from build123d import *

# Parameters (mm, degrees)
BOSS_EXTRUDE1_DEPTH = 5
CUT_EXTRUDE2_DEPTH  = 714.328929729


with BuildPart() as part:
    # Sketch1 → Boss-Extrude1 (new body)
    with BuildSketch(Plane(origin=(-68.393987025, -9.003975274, 13.699403605), x_dir=(0.23308919144115517, -0.5341135383088325, 0.8126451605888809), z_dir=(0.972455360843524, 0.1280224242624249, -0.19478406005796045))):
        Polygon((290.734459145, 269.471566891), (290.734459145, 334.44233671), (415.531866377, 494.175733816), (509.260454317, 494.175733816), (509.260454317, 469.175733816), (446.760454317, 469.175733816), align=None)
    extrude(amount=BOSS_EXTRUDE1_DEPTH)

    # Sketch3 → Cut-Extrude2 (cut, through all)
    with BuildSketch(Plane(origin=(-63.53171022, -8.363863152, 12.725483305), x_dir=(-0.193117751863984, -0.025423689104136546, -0.9808461499885377), z_dir=(0.9724553608435241, 0.1280224242624253, -0.19478406005796034))):
        Polygon((-103.20824521, -577.778495346), (-102.919185311, -573.588454251), (-98.928669982, -573.863749393), (-98.811669547, -572.167780379), (-96.018308817, -572.360486979), (-96.135309253, -574.056455993), (-86.159020932, -574.74469385), (-86.448080832, -578.934734944), (-96.424369152, -578.246497088), (-96.541369588, -579.942466102), (-99.334730318, -579.749759503), (-99.217729882, -578.053790488), align=None)
        Polygon((-94.487300279, -451.364843062), (-94.19824038, -447.174801967), (-90.207725052, -447.45009711), (-90.090724616, -445.754128095), (-87.297363886, -445.946834695), (-87.414364322, -447.64280371), (-77.438076001, -448.331041566), (-77.727135901, -452.521082661), (-87.703424221, -451.832844804), (-87.820424657, -453.528813819), (-90.613785387, -453.336107219), (-90.496784951, -451.640138205), align=None)
        Polygon((-130.671777813, -684.777132582), (-134.151538298, -687.128997155), (-136.39140932, -683.81493955), (-137.799883802, -684.766884734), (-139.367793517, -682.447044411), (-137.959319035, -681.495099227), (-143.558996589, -673.209955215), (-140.079236104, -670.858090643), (-134.47955855, -679.143234654), (-133.071084068, -678.19128947), (-131.503174353, -680.511129793), (-132.911648835, -681.463074978), align=None)
    extrude(amount=-CUT_EXTRUDE2_DEPTH, mode=Mode.SUBTRACT)


solid = part.part
CAD build for the part. Positions are in the model's coordinates, mm. A direction names the side the tool comes from. Round coordinates to 2 decimals unless told otherwise and drop trailing zeros. Loops run counter-clockwise (first coordinate to the right, second up) from the corner with the lowest first, then second, coordinate; pieces in that order, holes last. Notation, with made-up numbers: (32, -11) - (47, -11) arc R21 cw to (47, 21) - close; hole circle Ø7 at (-27.75, 44.5). An arc over 180 degrees is marked (long way). Put each result on its own line as item: value.
1. Pin check, flat tips, straight feed: P1, Ø4, axis at y = -491, z = 110.5, coming from the -X side; P2, Ø8, axis at y = -663, z = 96.5, coming from the +X side; P3, Ø10, axis at y = -466.5, z = 76.5, coming from the -X side; P4, Ø1, axis at y = -475, z = 101.5, coming from the -X side. Stop position of each tip, or through.
Geometry check:
P1: x = 13.97
P2: through
P3: x = 3.22
P4: x = 10.42
2. Wall check: line 1 (X direction, y = -611, z = 101); line 2 (X direction, y = -441.5, z = 70.5). Give the ranges that are in metal, low to high.
Geometry check:
line 1: 28.34 to 33.49
line 2: -0.08 to 5.06
3. Slice it at B-B on y = -654. List the corners of the cut face in (x, z), and give its area (3 significant figures).
Geometry check:
outline: (32.87, 95.31) - (38.01, 95.31) - (47.12, 140.83) - (41.98, 140.83) - close
area: 234 mm²
4. 3-axis set-ups, long thin cutter, end or side, ignore diameter. For faces 4 (the flat face through (48.69, -674.36, 147.89)), 5 (the flat face through (49.66, -676.72, 151.23)), 6 (the flat face through (8.474, -450.732, 94.122)): which of +Z, -Z, +X, -X, +Y, -Y reach the whole face in a straight line?
Geometry check:
face 4: +X
face 5: -X
face 6: +Z, +X
5. Two-plate mould, pull along Z, no slides. Class faces 1 (the flat face through (6.227, -419.825, 103.575)), 2 (the flat face through (51.129, -690.042, 150.147)), 3 (the flat face through (9.05, -454.89, 94.27)): released by +Z, released by -Z, zero draft, split by the parting line, or undercut.
Geometry check:
face 1: released by +Z
face 2: released by -Z
face 3: undercut
6. Slice it at A-A on z = 74. List the corners of the cut face in (x, y), and give its area (3 significant figures).
Geometry check:
outline: (-0.63, -432.01) - (15.8, -556.78) - (22.73, -570.38) - (4.24, -429.89) - close
area: 682 mm²
